Part model, mm, in its own coordinate system. Face numbers are marked on the shaded views. A direction names the side the tool comes from. Round coordinates to 2 decimals unless told otherwise and drop trailing zeros. Loops run counter-clockwise (first coordinate to the right, second up) from the corner with the lowest first, then second, coordinate; pieces in that order, holes last. Notation, with made-up numbers: (43.5, 83.5) -> (56.5, 83.5) arc R26 ccw to (56.5, 110.5) -> close; hole circle Ø6 at (15, 28). An arc over 180 degrees is marked (long way). Answer as a JSON object with one key per item and string values. Group by question number.
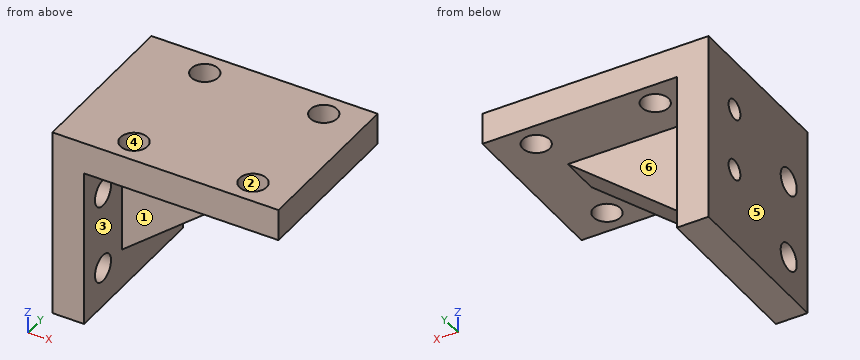
from build123d import *

# Parameters (mm, degrees)
SKETCH_1_W          = 28.5
SKETCH_1_H          = 21
EXTRUDE_1_DEPTH     = 4
SKETCH_2_W          = 4
SKETCH_2_H          = 21
EXTRUDE_2_DEPTH     = 20
RIB_1_REACH         = 38.366
SKETCH_3_WALL_W     = 98.549396912
SKETCH_3_WALL_H     = 5
CUT_EXTRUDE_1_REACH = 42.66
SKETCH_4_R          = 1.25
CUT_EXTRUDE_2_REACH = 44.77
SKETCH_5_R          = 1.7
CUT_EXTRUDE_3_REACH = 39.964
SKETCH_6_R          = 1.7


with BuildPart() as part:
    # 草图1 → 凸台-拉伸1 (new body)
    with BuildSketch(Plane.XY):
        with Locations((14.25, 10.5)):
            Rectangle(SKETCH_1_W, SKETCH_1_H)
    extrude(amount=EXTRUDE_1_DEPTH)

    # 草图2 → 凸台-拉伸2 (add)
    with BuildSketch(Plane(origin=(0, 0, 0), x_dir=(-1, 0, 0), z_dir=(0, 0, -1))):
        with Locations((-2, 10.5)):
            Rectangle(SKETCH_2_W, SKETCH_2_H)
    extrude(amount=EXTRUDE_2_DEPTH)

    # 草图3 wall → 筋1 (add, up to next)
    with BuildSketch(Plane(origin=(13.25, 10.5, -7.5), x_dir=(-0.77675574872, 0, -0.629801958421), z_dir=(0.629801958421, 0, -0.77675574872)), mode=Mode.PRIVATE) as rib_1_sk1:
        Rectangle(SKETCH_3_WALL_W, SKETCH_3_WALL_H)
    rib_1_tool1 = extrude(rib_1_sk1.sketch, amount=-RIB_1_REACH, mode=Mode.PRIVATE) - part.part
    add(rib_1_tool1.solids().sort_by_distance((13.25, 10.5, -7.5))[0])

    # 草图4 → 切除-拉伸1 (cut, up to next)
    with BuildSketch(Plane.ZY, mode=Mode.PRIVATE) as cut_extrude_1_sk1:
        with Locations((-2.406007896, 15.5)):
            Circle(SKETCH_4_R)
    cut_extrude_1_tool1 = extrude(cut_extrude_1_sk1.sketch, amount=-CUT_EXTRUDE_1_REACH, mode=Mode.PRIVATE) & part.part
    # 草图4 → 切除-拉伸1 (cut, up to next)
    with BuildSketch(Plane.ZY, mode=Mode.PRIVATE) as cut_extrude_1_sk2:
        with Locations((-10.406007896, 15.5)):
            Circle(SKETCH_4_R)
    cut_extrude_1_tool2 = extrude(cut_extrude_1_sk2.sketch, amount=-CUT_EXTRUDE_1_REACH, mode=Mode.PRIVATE) & part.part
    add(cut_extrude_1_tool1.solids().sort_by_distance((0, 15.5, -2.406008))[0], mode=Mode.SUBTRACT)
    add(cut_extrude_1_tool2.solids().sort_by_distance((0, 15.5, -10.406008))[0], mode=Mode.SUBTRACT)

    # 草图5 → 切除-拉伸2 (cut, up to next)
    with BuildSketch(Plane.XY.offset(4), mode=Mode.PRIVATE) as cut_extrude_2_sk1:
        with Locations((23.5, 18)):
            Circle(SKETCH_5_R)
    cut_extrude_2_tool1 = extrude(cut_extrude_2_sk1.sketch, amount=-CUT_EXTRUDE_2_REACH, mode=Mode.PRIVATE) & part.part
    # 草图5 → 切除-拉伸2 (cut, up to next)
    with BuildSketch(Plane.XY.offset(4), mode=Mode.PRIVATE) as cut_extrude_2_sk2:
        with Locations((8.5, 3)):
            Circle(SKETCH_5_R)
    cut_extrude_2_tool2 = extrude(cut_extrude_2_sk2.sketch, amount=-CUT_EXTRUDE_2_REACH, mode=Mode.PRIVATE) & part.part
    # 草图5 → 切除-拉伸2 (cut, up to next)
    with BuildSketch(Plane.XY.offset(4), mode=Mode.PRIVATE) as cut_extrude_2_sk3:
        with Locations((23.5, 3)):
            Circle(SKETCH_5_R)
    cut_extrude_2_tool3 = extrude(cut_extrude_2_sk3.sketch, amount=-CUT_EXTRUDE_2_REACH, mode=Mode.PRIVATE) & part.part
    # 草图5 → 切除-拉伸2 (cut, up to next)
    with BuildSketch(Plane.XY.offset(4), mode=Mode.PRIVATE) as cut_extrude_2_sk4:
        with Locations((8.5, 18)):
            Circle(SKETCH_5_R)
    cut_extrude_2_tool4 = extrude(cut_extrude_2_sk4.sketch, amount=-CUT_EXTRUDE_2_REACH, mode=Mode.PRIVATE) & part.part
    add(cut_extrude_2_tool1.solids().sort_by_distance((23.5, 18, 4))[0], mode=Mode.SUBTRACT)
    add(cut_extrude_2_tool2.solids().sort_by_distance((8.5, 3, 4))[0], mode=Mode.SUBTRACT)
    add(cut_extrude_2_tool3.solids().sort_by_distance((23.5, 3, 4))[0], mode=Mode.SUBTRACT)
    add(cut_extrude_2_tool4.solids().sort_by_distance((8.5, 18, 4))[0], mode=Mode.SUBTRACT)

    # 草图6 → 切除-拉伸3 (cut, up to next)
    with BuildSketch(Plane(origin=(4, 0, 0), x_dir=(0, 0, -1), z_dir=(1, 0, 0)), mode=Mode.PRIVATE) as cut_extrude_3_sk1:
        with Locations((5, 4)):
            Circle(SKETCH_6_R)
    cut_extrude_3_tool1 = extrude(cut_extrude_3_sk1.sketch, amount=-CUT_EXTRUDE_3_REACH, mode=Mode.PRIVATE) & part.part
    # 草图6 → 切除-拉伸3 (cut, up to next)
    with BuildSketch(Plane(origin=(4, 0, 0), x_dir=(0, 0, -1), z_dir=(1, 0, 0)), mode=Mode.PRIVATE) as cut_extrude_3_sk2:
        with Locations((15, 4)):
            Circle(SKETCH_6_R)
    cut_extrude_3_tool2 = extrude(cut_extrude_3_sk2.sketch, amount=-CUT_EXTRUDE_3_REACH, mode=Mode.PRIVATE) & part.part
    add(cut_extrude_3_tool1.solids().sort_by_distance((4, 4, -5))[0], mode=Mode.SUBTRACT)
    add(cut_extrude_3_tool2.solids().sort_by_distance((4, 4, -15))[0], mode=Mode.SUBTRACT)


solid = part.part
Item 1: Band-saw the part on D-D, the plane y = 3. List the corners of the cut face in (x, z), plus the area to 3 significant figures.
Item 2: Band-saw the part on A-A, the plane y = 15.5. List the corners of the cut face in (x, z).
Item 3: Drill centre lines: line 1 (Y direction, x = 8.5, z = 2.45); line 2 (Z direction, x = 17.25, y = 4.5); line 3 (Y direction, x = 4.25, z = -9). Where is each one in solid material? Low to high.
Item 4: Drop flat-ended pins along their axis: pin 1 Ø12 at (x, z) = (11, -9.5) entering from -Y; pin 2 Ø4 at (y, z) = (4, -5) entering from +X; pin 3 Ø8 at (y, z) = (14.5, -16.5) entering from +X. Give the stop position or say it passes through.
Item 5: Band-saw the part on C-C, the plane x = 8.5. List the corners of the cut face in (y, z), plus the area to 3 significant figures.
Item 6: Band-saw the part on B-B, the plane z = -11.25. List the corners of the cut face in (x, y) (3 decimals), plus the area to 3 significant figures.
Item 7: Two-plate mould, pull along Y, no slides. Class the marked faces 4, 5 and 6: pulls with the +Y half, pulls with the -Y half, needs draft (parallel to the pull), parting line crosses it, or undercut.
Item 8: Which spindle directions (+Z, -Z, +X, -X, +Y, -Y) get a long thin tool onto all of the face, cutting with end or side? Do the marked faces 1, 2 and 3. Say none if no direction does.
Entries:
{
 "1": {"outline": "(0, -20) -> (4, -20) -> (4, -16.37) -> (0, -16.37) -> close; (0, -13.63) -> (4, -13.63) -> (4, -6.37) -> (0, -6.37) -> close; (0, -3.63) -> (4, -3.63) -> (4, 0) -> (6.8, 0) -> (6.8, 4) -> (0, 4) -> close; (10.2, 0) -> (21.8, 0) -> (21.8, 4) -> (10.2, 4) -> close; (25.2, 0) -> (28.5, 0) -> (28.5, 4) -> (25.2, 4) -> close", "area": "145 mm²"},
 "2": {"outline": "(0, -20) -> (4, -20) -> (4, -11.66) -> (0, -11.66) -> close; (0, -9.16) -> (4, -9.16) -> (4, -3.66) -> (0, -3.66) -> close; (0, -1.16) -> (4, -1.16) -> (4, 0) -> (28.5, 0) -> (28.5, 4) -> (0, 4) -> close"},
 "3": {"line 1": "0 to 1.3, 4.7 to 16.3, 19.7 to 21", "line 2": "0 to 4", "line 3": "8 to 13"},
 "4": {"pin 1": "y = 8", "pin 2": "x = 4", "pin 3": "x = 6.72"},
 "5": {"outline": "(0, 0) -> (1.3, 0) -> (1.3, 4) -> (0, 4) -> close; (4.7, 0) -> (8, 0) -> (8, -11.35) -> (13, -11.35) -> (13, 0) -> (16.3, 0) -> (16.3, 4) -> (4.7, 4) -> close; (19.7, 0) -> (21, 0) -> (21, 4) -> (19.7, 4) -> close", "area": "114 mm²"},
 "6": {"outline": "(0, 0) -> (4, 0) -> (4, 8) -> (8.625, 8) -> (8.625, 13) -> (4, 13) -> (4, 14.578) -> (0, 14.578) -> close; (0, 16.422) -> (4, 16.422) -> (4, 21) -> (0, 21) -> close", "area": "99.7 mm²"},
 "7": {"face 4": "undercut", "face 5": "needs draft", "face 6": "pulls with the +Y half"},
 "8": {"face 1": "-Z, +X, -Y", "face 2": "+Z, -Z", "face 3": "-Z, +X"}
}
